```python
from build123d import *

# Parameters (mm, degrees)
EXTRUDE_1_DEPTH     = 20
CUT_EXTRUDE_1_DEPTH = 10
SKETCH_3_R          = 21
CUT_EXTRUDE_2_DEPTH = 8
SKETCH_6_R          = 1.5
CUT_EXTRUDE_3_DEPTH = 5
SKETCH_7_R          = 1.5
CUT_EXTRUDE_6_DEPTH = 3
SKETCH_8_R          = 6
CUT_EXTRUDE_7_DEPTH = 3
SKETCH_9_W          = 10
SKETCH_9_H          = 20
SKETCH_9_R          = 1.5
EXTRUDE_2_DEPTH     = 3


with BuildPart() as part:
    # 草图1 → 凸台-拉伸1 (new body)
    with BuildSketch(Plane.XY):
        with BuildLine():
            Line((-23, 0), (-23, -27))
            Line((-23, -27), (23, -27))
            Line((23, -27), (23, 0))
            ThreePointArc((23, 0), (0, 23), (-23, 0))
        make_face()
    extrude(amount=EXTRUDE_1_DEPTH)

    # 草图2 → 切除-拉伸1 (cut)
    with BuildSketch(Plane(origin=(0, 0, 0), x_dir=(-1, 0, 0), z_dir=(0, 0, -1))):
        with BuildLine():
            Line((-23, -24), (23, -24))
            Line((23, -24), (23, 0))
            ThreePointArc((23, 0), (0, 23), (-23, 0))
            Line((-23, 0), (-23, -24))
        make_face()
    extrude(amount=-CUT_EXTRUDE_1_DEPTH, mode=Mode.SUBTRACT)

    # 草图3 → 切除-拉伸2 (cut)
    with BuildSketch(Plane(origin=(0, 0, 10), x_dir=(-1, 0, 0), z_dir=(0, 0, -1))):
        Circle(SKETCH_3_R)
    extrude(amount=-CUT_EXTRUDE_2_DEPTH, mode=Mode.SUBTRACT)

    # 草图6 → 切除-拉伸3 (cut)
    with BuildSketch(Plane.XZ.offset(27)):
        with Locations(Location((-18, 15, 0), (0, 0, 270))):
            Circle(SKETCH_6_R)
        with Locations(Location((18, 15, 0), (0, 0, 90))):
            Circle(SKETCH_6_R)
        with Locations(Location((18, 5, 0), (0, 0, 270))):
            Circle(SKETCH_6_R)
        with Locations(Location((-18, 5, 0), (0, 0, 270))):
            Circle(SKETCH_6_R)
    extrude(amount=-CUT_EXTRUDE_3_DEPTH, mode=Mode.SUBTRACT)

    # 草图7 → 切除-拉伸6 (cut)
    with BuildSketch(Plane.XY.offset(20)):
        with Locations((0, 16)):
            Circle(SKETCH_7_R)
        with Locations((12.589057749, 9.875)):
            Circle(SKETCH_7_R)
        with Locations((-12.589057749, -9.875)):
            Circle(SKETCH_7_R)
        with Locations((15.539618159, -3.810546875)):
            Circle(SKETCH_7_R)
    extrude(amount=-CUT_EXTRUDE_6_DEPTH, mode=Mode.SUBTRACT)

    # 草图8 → 切除-拉伸7 (cut)
    with BuildSketch(Plane(origin=(0, 0, 18), x_dir=(-1, 0, 0), z_dir=(0, 0, -1))):
        Circle(SKETCH_8_R)
    extrude(amount=-CUT_EXTRUDE_7_DEPTH, mode=Mode.SUBTRACT)

    # 草图9 → 凸台-拉伸2 (add)
    # profile 1 of 2: a face of its own
    with BuildSketch(Plane.XZ.offset(27)):
        with Locations((28, 10)):
            Rectangle(SKETCH_9_W, SKETCH_9_H)
        with Locations(Location((28, 15, 0), (0, 0, 270))):
            Circle(SKETCH_9_R, mode=Mode.SUBTRACT)
        with Locations(Location((28, 5, 0), (0, 0, 270))):
            Circle(SKETCH_9_R, mode=Mode.SUBTRACT)
    # profile 2 of 2: a face of its own
    with BuildSketch(Plane.XZ.offset(27)):
        with Locations((-28, 10)):
            Rectangle(SKETCH_9_W, SKETCH_9_H)
        with Locations(Location((-28, 15, 0), (0, 0, 90))):
            Circle(SKETCH_9_R, mode=Mode.SUBTRACT)
        with Locations(Location((-28, 5, 0), (0, 0, 90))):
            Circle(SKETCH_9_R, mode=Mode.SUBTRACT)
    extrude(amount=-EXTRUDE_2_DEPTH)


solid = part.part
```
The model under review builds one solid part; all positions refer to its coordinate system, in mm. A direction names the side the tool comes from. Round coordinates to 2 decimals unless told otherwise and drop trailing zeros. Write each loop counter-clockwise with the first axis right and the second up, starting at its lowest first coordinate (ties: lowest second). Pieces come first, ordered by that corner, then holes. Notation, with made-up numbers: M -9,17.5 L 9,17.5 A32 cw 9,55.5 Z; hole C 3.25,-24.5 d4. An arc over 180 degrees is marked long. Use CSV: the item, a comma, the result in double quotes. Start each with the question number.
(1) Clearance check with flat-ended pins moving along their axes: P1, Ø2, axis at x = -8.5, z = 7, coming from the +Y side; P2, Ø1.5, axis at x = -18.5, z = 15.5, coming from the -Y side; P3, Ø2.5, axis at x = 18, z = 15, coming from the +Y side. State where each tip first meets the part, or that it passes through.
(2) Tool access review of faces 5 (the face through (18, -22, 15)), 6 (the face through (0.1, -21.3, 10)), 7 (the face through (-20.03, 6.31, 13.94)), 8 (the face through (-23, -12, 15)): name each direction out of +Z, -Z, +X, -X, +Y, -Y from which nothing blocks a thin tool from reaching the whole face with its end or side.
(3) We need section A-A, the plane z = 5. State the section outline as (x, y) points.
(4) We need section C-C, the plane y = 16. State the section outline as (x, z) points, then the cut area to 3 significant figures.
(5) We need section D-D, the plane z = 15.5. State the section outline as (x, y) points.
(6) For line 1 along Y through (x, z) = (0, 19.25); line 2 along X through (y, z) = (-24.75, 5); line 3 along Z through (x, y) = (19, -21), list the stretches that pass through material, from the lowest coordinate up.
(7) We need section B-B, the plane x = 0. State the section outline as (y, z) points, then the cut area to 3 significant figures.
(8) The part is to be moulded in two halves that separate along X. For faces 1 (the face through (0, -26, 0)), 2 (the face through (33, -26, 10)), 3 (the face through (-16.99, -24.54, 16.11)), 4 (the face through (19.487, -25.521, 5.195)), say which applies: +X half, -X half, draft (parallel to the pull), parting line (faces both ways), or undercut.
Findings:
1,P1,"y = -24"
1,P2,"y = -22"
1,P3,"y = 15.76"
2,face 5,"-Y"
2,face 6,"-Z, +X, -X, +Y"
2,face 7,"-Z"
2,face 8,"+Z, -Z, -X, +Y"
3,outline,"M -33,-27 L -29.5,-27 L -29.5,-24 L -33,-24 Z; M -26.5,-27 L -19.5,-27 L -19.5,-24 L -26.5,-24 Z; M -16.5,-27 L 16.5,-27 L 16.5,-24 L -16.5,-24 Z; M 19.5,-27 L 26.5,-27 L 26.5,-24 L 19.5,-24 Z; M 29.5,-27 L 33,-27 L 33,-24 L 29.5,-24 Z"
4,outline,"M -16.52,10 L -13.6,10 L -13.6,18 L -1.5,18 L -1.5,20 L -16.52,20 Z; M 1.5,18 L 13.6,18 L 13.6,10 L 16.52,10 L 16.52,20 L 1.5,20 Z"
4,area,"107 mm^2"
5,outline,"M -33,-27 L -29.41,-27 L -29.41,-24 L -33,-24 Z; M -26.59,-27 L -19.41,-27 L -19.41,-22 L -16.59,-22 L -16.59,-27 L 16.59,-27 L 16.59,-22 L 19.41,-22 L 19.41,-27 L 26.59,-27 L 26.59,-24 L 23,-24 L 23,0 A23 ccw -23,0 L -23,-24 L -26.59,-24 Z; M 29.41,-27 L 33,-27 L 33,-24 L 29.41,-24 Z; hole C 0,0 d42"
6,line 1,"-27 to -6, 6 to 14.5, 17.5 to 23"
6,line 2,"-33 to -29.5, -26.5 to -19.5, -16.5 to 16.5, 19.5 to 26.5, 29.5 to 33"
6,line 3,"10 to 20"
7,outline,"M -27,0 L -24,0 L -24,10 L -21,10 L -21,18 L -6,18 L -6,20 L -27,20 Z; M 6,18 L 14.5,18 L 14.5,20 L 6,20 Z; M 17.5,18 L 21,18 L 21,10 L 23,10 L 23,20 L 17.5,20 Z"
7,area,"164 mm^2"
8,face 1,"draft"
8,face 2,"+X half"
8,face 3,"undercut"
8,face 4,"undercut"
